Source: CAD feature listing. Evaluate the final solid. Frame: model axes, mm. A direction names the side the tool comes from. Give positions to 0.01 mm unless a question says otherwise; leave off trailing zeros. Order: outer loops, then holes, each group sorted by start corner. A loop starts at its lowest first (then second) coordinate and runs counter-clockwise, first axis right, second up. Notation, with made-up numbers: (5, -13.75) - (46, -13.75) arc R14 ccw to (46, -9.75) - close; hole circle Ø2 at (-37, 5.25). An arc over 180 degrees is marked (long way). Use CSV: the item, a comma, the result in double quotes.
```python
from build123d import *

# Parameters (mm, degrees)
RESSALTO_EXTRUS_O1_START         = 0.25
ESBO_O2_W                        = 30.5
ESBO_O2_H                        = 24.5
RESSALTO_EXTRUS_O1_DEPTH         = 3
ESBO_O3_W                        = 8.6
ESBO_O3_H                        = 24.5
RESSALTO_EXTRUS_O2_DEPTH         = 3
ESBO_O5_R                        = 4.25
CORTE_EXTRUS_O1_DEPTH            = 2
ESBO_O12_R                       = 3.5
CORTE_EXTRUS_O3_DEPTH            = 41.141904539
CBORE_FOR_M2_5_SHCS1_D           = 2.9
CBORE_FOR_M2_5_SHCS1_DEPTH       = 3
CBORE_FOR_M2_5_SHCS1_CBORE_D     = 5.5
CBORE_FOR_M2_5_SHCS1_CBORE_DEPTH = 2
FILETE1_R                        = 1.5


with BuildPart() as part:
    # Esboço2 → Ressalto-extrusão1 (new body)
    with BuildSketch(Plane.XY.offset(RESSALTO_EXTRUS_O1_START)):
        with Locations((15, -9.25)):
            Rectangle(ESBO_O2_W, ESBO_O2_H)
    extrude(amount=RESSALTO_EXTRUS_O1_DEPTH)

    # Esboço3 → Ressalto-extrusão2 (add)
    with BuildSketch(Plane.ZY.offset(0.25)):
        with Locations((-1.05, -9.25)):
            Rectangle(ESBO_O3_W, ESBO_O3_H)
    ressalto_extrus_o2 = extrude(amount=RESSALTO_EXTRUS_O2_DEPTH)

    # Espelhar1: Ressalto-extrusão2 across plane
    add(ressalto_extrus_o2.mirror(Plane.ZY.offset(-15)))

    # Esboço5 → Corte-extrusão1 (cut)
    with BuildSketch(Plane.XY.offset(3.25)):
        with Locations((15, -6)):
            Circle(ESBO_O5_R)
    extrude(amount=-CORTE_EXTRUS_O1_DEPTH, mode=Mode.SUBTRACT)

    # Esboço12 → Corte-extrusão3 (cut, through all)
    with BuildSketch(Plane.XY.offset(1.25)):
        with Locations((15, -6)):
            Circle(ESBO_O12_R)
    extrude(amount=-CORTE_EXTRUS_O3_DEPTH, mode=Mode.SUBTRACT)

    # CBORE for M2.5 SHCS1
    with Locations(Plane.ZY.offset(3.25)):
        with Locations((-2.8, -1.5), (-2.8, -18.5)):
            cbore_for_m2_5_shcs1 = CounterBoreHole(CBORE_FOR_M2_5_SHCS1_D / 2, CBORE_FOR_M2_5_SHCS1_CBORE_D / 2, CBORE_FOR_M2_5_SHCS1_CBORE_DEPTH, depth=CBORE_FOR_M2_5_SHCS1_DEPTH)

    # Mirror1: CBORE for M2.5 SHCS1 across plane
    add(cbore_for_m2_5_shcs1.mirror(Plane.ZY.offset(-15)), mode=Mode.SUBTRACT)

    # Filete1
    filete1_edges = [part.edges().sort_by_distance(p)[0] for p in [
        (-3.25, -9.25, 3.25),
        (33.25, -9.25, 3.25),
    ]]
    fillet(filete1_edges, radius=FILETE1_R)


solid = part.part
```
Item 1: Set-up query: faces 1 (the flat face through (32, -9, -5.35)), 2 (the cylindrical face through (14.447, -1.786, 2.264)), 3 (the flat face through (30.25, -9, -3)), 4 (the flat face through (31.25, -20, -4)), 5 (the flat face through (-1.25, -20, -4)). Return all of +Z, -Z, +X, -X, +Y, -Y with unobstructed straight access to the full face (end or side cutting, diameter ignored); none if empty.
Filled in:
face 1,"-Z, +X, -X, +Y, -Y"
face 2,"+Z"
face 3,"-Z, +Y, -Y"
face 4,"+X"
face 5,"-X"
Item 2: Section A-A on y = -15. Return the cut outline in (x, z), then the cut area to 3 significant figures.
Filled in:
outline,"(-3.25, -5.35) - (-0.25, -5.35) - (-0.25, 0.25) - (30.25, 0.25) - (30.25, -5.35) - (33.25, -5.35) - (33.25, 1.75) arc R1.5 ccw to (31.75, 3.25) - (-1.75, 3.25) arc R1.5 ccw to (-3.25, 1.75) - close"
area,"142 mm2"
Item 3: Mould query, pull axis Z, two halves, no side actions, for faces 6 (the cylindrical face through (-0.74, -0.52, -1.73)), 7 (the cylindrical face through (32.8, -9.08, 2.82)), 8 (the flat face through (-3.25, -9, -1)). Classes: released by +Z, released by -Z, zero draft, split by the parting line, or undercut.
Filled in:
face 6,"undercut"
face 7,"released by +Z"
face 8,"zero draft"
Item 4: Material intervals for line 1 (Y direction, x = -0.85, z = -2.8); line 2 (X direction, y = -14.75, z = -0.5); line 3 (X direction, y = 0.5, z = -3.25), sorted ascending. Write a range as from..to.
Filled in:
line 1,"y = -21.5..-19.95, -17.05..-2.95, -0.05..3"
line 2,"x = -3.25..-0.25, 30.25..33.25"
line 3,"x = -1.25..-0.25, 30.25..31.25"
Item 5: Section B-B on x = 15.5. Return the cut outline in (y, z).
Filled in:
outline,"(-21.5, 0.25) - (-9.46, 0.25) - (-9.46, 1.25) - (-10.22, 1.25) - (-10.22, 3.25) - (-21.5, 3.25) - close; (-2.54, 0.25) - (3, 0.25) - (3, 3.25) - (-1.78, 3.25) - (-1.78, 1.25) - (-2.54, 1.25) - close"
Item 6: First-contact query: pin 1 (4.5 mm diameter, centred on y = -18.5, z = -2.8, fed in from -X); pin 2 (2 mm diameter, centred on x = 16.5, z = 0, fed in from -Y); pin 3 (12 mm diameter, centred on x = 22.5, y = -7, fed in from -Z); pin 4 (4 mm diameter, centred on x = 14.5, y = -8, fed in from +Z). Flat tips, straight axial feed; report the tip coordinate or a pass-through.
Filled in:
pin 1,"stops at x = -1.25"
pin 2,"stops at y = -21.5"
pin 3,"stops at z = 0.25"
pin 4,"stops at z = 1.25"
Item 7: Section C-C on z = -2.8. Count the separate pieces of the cut face and the enclosed holes in it, then the cut area to 3 significant figures.
Filled in:
separate pieces,"6"
enclosed holes,"0"
area,"91.4 mm2"
Item 8: Section D-D on y = -8.5. Return the cut outline in (x, z).
Filled in:
outline,"(-3.25, -5.35) - (-0.25, -5.35) - (-0.25, 0.25) - (12.55, 0.25) - (12.55, 1.25) - (11.56, 1.25) - (11.56, 3.25) - (-1.75, 3.25) arc R1.5 ccw to (-3.25, 1.75) - close; (17.45, 0.25) - (30.25, 0.25) - (30.25, -5.35) - (33.25, -5.35) - (33.25, 1.75) arc R1.5 ccw to (31.75, 3.25) - (18.44, 3.25) - (18.44, 1.25) - (17.45, 1.25) - close"
